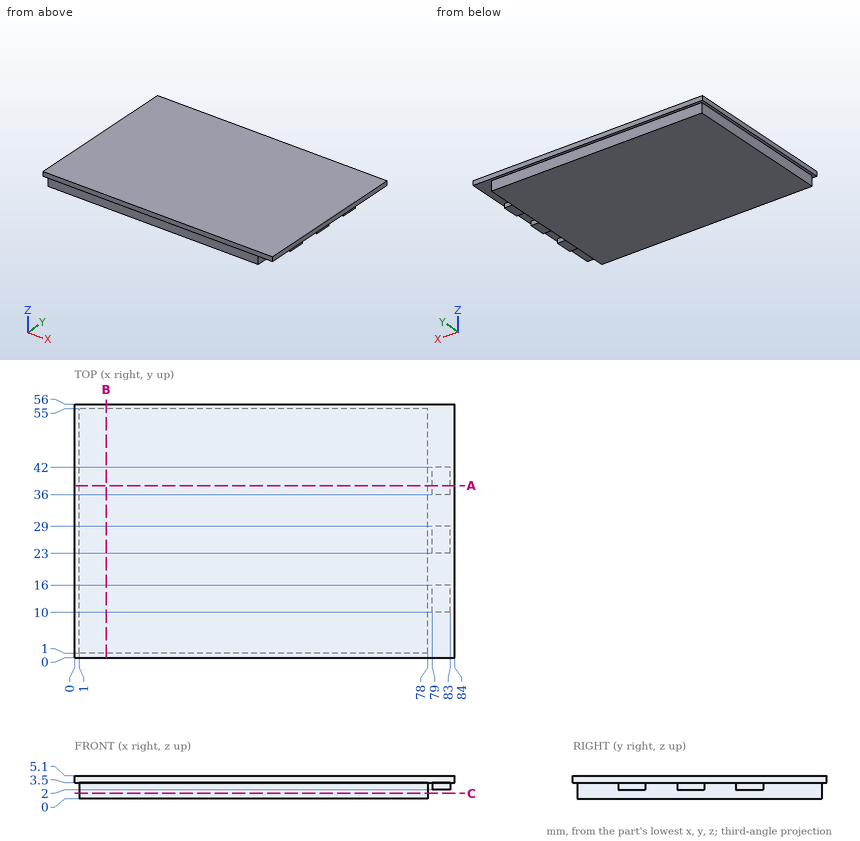
For this review, use the dimensioned drawing (mm, ordinates from the lowest corner) and the shaded views. Round coordinates to 2 decimals unless told otherwise and drop trailing zeros. Write each loop counter-clockwise with the first axis right and the second up, starting at its lowest first coordinate (ties: lowest second). Pieces come first, ordered by that corner, then holes. Notation, with made-up numbers: (-36.5, -31) - (-16.5, -31) arc R15 cw to (-16.5, -15) - close; hole circle Ø9 at (9, 34.5). An arc over 180 degrees is marked (long way). Use CSV: the item, a comma, the result in double quotes.
1) Add section C-C on z = 1.15. Write out the cut boundary in (x, y).
Conclusion:
outline,"(1, 1) - (78, 1) - (78, 55) - (1, 55) - close"
2) Add section A-A on y = 38. Write out the cut boundary in (x, z), and give its area (3 significant figures).
Conclusion:
outline,"(0, 3.5) - (1, 3.5) - (1, 0) - (78, 0) - (78, 3.5) - (79, 3.5) - (79, 2) - (83, 2) - (83, 3.5) - (84, 3.5) - (84, 5.1) - (0, 5.1) - close"
area,"410 mm^2"
3) Wall thickness on line 1 along X through (y, z) = (12.5, 3.25); line 2 along X through (y, z) = (43, 1.45); line 3 along Y through (x, z) = (32.5, 2.7): over which ranges is each line inside the solid? List them lowest first. Write a range as from..to.
Conclusion:
line 1,"x = 1..78, 79..83"
line 2,"x = 1..78"
line 3,"y = 1..55"
4) Add section B-B on x = 7. Write out the cut boundary in (y, z).
Conclusion:
outline,"(0, 3.5) - (1, 3.5) - (1, 0) - (55, 0) - (55, 3.5) - (56, 3.5) - (56, 5.1) - (0, 5.1) - close"
5) Clearance check with flat-ended pins moving along their axes: pin 1 Ø1.2 at (y, z) = (27.5, 2.5) entering from -X; pin 2 Ø1.6 at (x, z) = (81, 3) entering from -Y; pin 3 Ø1.2 at (x, z) = (80, 2.5) entering from +Y; pin 4 Ø2 at (x, y) = (81.5, 40.5) entering from -Z. State where each tip first meets the part, or that it passes through.
Conclusion:
pin 1,"stops at x = 1"
pin 2,"stops at y = 0"
pin 3,"stops at y = 42"
pin 4,"stops at z = 2"
